from build123d import *

# Parameters (mm, degrees)
SKETCH2_W           = 120.65
SKETCH2_H           = 120.65
BOSS_EXTRUDE1_DEPTH = 2.54
SKETCH3_W           = 52.07
SKETCH3_H           = 16.51
SKETCH3_W_2         = 0.635
SKETCH3_H_2         = 6.35
SKETCH3_H_3         = 27.94
SKETCH3_W_3         = 23.495
SKETCH3_H_4         = 38.1
BOSS_EXTRUDE2_DEPTH = 2.54
BOSS_EXTRUDE4_DEPTH = 2.54


with BuildPart() as part:
    # Sketch2 → Boss-Extrude1 (new body)
    with BuildSketch(Plane(origin=(0, 0, 0), x_dir=(1, 0, 0), z_dir=(0, 1, 0))):
        Rectangle(SKETCH2_W, SKETCH2_H)
    extrude(amount=BOSS_EXTRUDE1_DEPTH)

    # Sketch3 → Boss-Extrude2 (add)
    with BuildSketch(Plane(origin=(0, 2.54, 0), x_dir=(1, 0, 0), z_dir=(0, 1, 0))):
        with Locations((-28.575, 52.07)):
            Rectangle(SKETCH3_W, SKETCH3_H)
        with Locations((-60.0075, -21.59)):
            Rectangle(SKETCH3_W_2, SKETCH3_H_2)
        with Locations((60.0075, -46.355)):
            Rectangle(SKETCH3_W_2, SKETCH3_H_3)
        with Locations((-42.8625, -21.59)):
            Rectangle(SKETCH3_W_3, SKETCH3_H_2)
        with Locations((-14.2875, -21.59)):
            Rectangle(SKETCH3_W_3, SKETCH3_H_2)
        with Locations((-60.0075, 52.07)):
            Rectangle(SKETCH3_W_2, SKETCH3_H)
        with Locations((60.0075, 5.715)):
            Rectangle(SKETCH3_W_2, SKETCH3_H_4)
        with Locations((42.8625, -21.59)):
            Rectangle(SKETCH3_W_3, SKETCH3_H_2)
        with Locations((14.2875, -21.59)):
            Rectangle(SKETCH3_W_3, SKETCH3_H_2)
        with Locations((-60.0075, 5.715)):
            Rectangle(SKETCH3_W_2, SKETCH3_H_4)
        with Locations((-60.0075, -46.355)):
            Rectangle(SKETCH3_W_2, SKETCH3_H_3)
        with Locations((60.0075, 52.07)):
            Rectangle(SKETCH3_W_2, SKETCH3_H)
        with Locations((28.575, 52.07)):
            Rectangle(SKETCH3_W, SKETCH3_H)
        with Locations((-28.575, -46.355)):
            Rectangle(SKETCH3_W, SKETCH3_H_3)
        with Locations((28.575, -46.355)):
            Rectangle(SKETCH3_W, SKETCH3_H_3)
        with Locations((60.0075, -21.59)):
            Rectangle(SKETCH3_W_2, SKETCH3_H_2)
        with Locations((28.575, 5.715)):
            Rectangle(SKETCH3_W, SKETCH3_H_4)
        with Locations((-42.8625, 35.56)):
            Rectangle(SKETCH3_W_3, SKETCH3_H_2)
        with Locations((-14.2875, 35.56)):
            Rectangle(SKETCH3_W_3, SKETCH3_H_2)
        with Locations((14.2875, 35.56)):
            Rectangle(SKETCH3_W_3, SKETCH3_H_2)
        with Locations((42.8625, 35.56)):
            Rectangle(SKETCH3_W_3, SKETCH3_H_2)
        with Locations((-28.575, 5.715)):
            Rectangle(SKETCH3_W, SKETCH3_H_4)
        with Locations((-60.0075, 35.56)):
            Rectangle(SKETCH3_W_2, SKETCH3_H_2)
        with Locations((60.0075, 35.56)):
            Rectangle(SKETCH3_W_2, SKETCH3_H_2)
    extrude(amount=BOSS_EXTRUDE2_DEPTH)

    # Sketch5 → Boss-Extrude4 (add)
    with BuildSketch(Plane(origin=(60.325, 0, 0), x_dir=(0, 0, -1), z_dir=(1, 0, 0))):
        Polygon((-60.325, 0), (60.325, 0), (60.325, 5.08), (43.815, 5.08), (43.815, 2.54), (38.735, 2.54), (38.735, 5.08), (32.385, 5.08), (32.385, 2.54), (24.765, 2.54), (24.765, 5.08), (-13.335, 5.08), (-13.335, 2.54), (-18.415, 2.54), (-18.415, 5.08), (-24.765, 5.08), (-24.765, 2.54), (-32.385, 2.54), (-32.385, 5.08), (-60.325, 5.08), align=None)
    boss_extrude4 = extrude(amount=BOSS_EXTRUDE4_DEPTH)

    # Mirror2: Boss-Extrude4 across plane
    add(boss_extrude4.mirror(Plane(origin=(0, 0, 0), x_dir=(0, 0, 1), z_dir=(1, 0, 0))))


solid = part.part
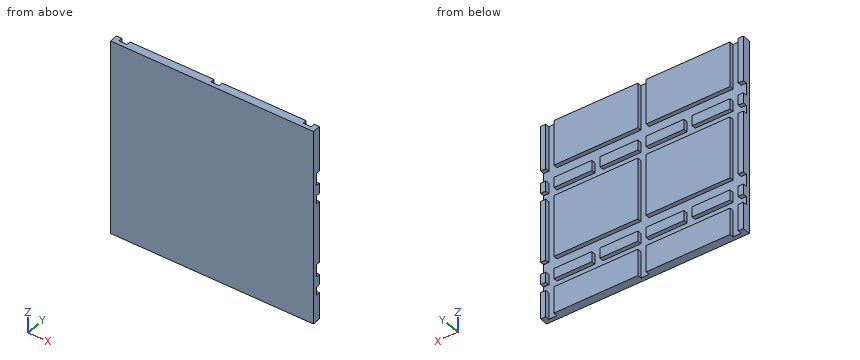
The model under review builds one solid part; all positions refer to its coordinate system, in mm. Coordinates: 2 decimals unless noted, no trailing zeros. Write each loop counter-clockwise with the first axis right and the second up, starting at its lowest first coordinate (ties: lowest second). Pieces come first, ordered by that corner, then holes. Notation, with made-up numbers: (53, 59.25) - (69, 59.25) arc R21 ccw to (69, 76.25) - close; hole circle Ø11 at (44.25, 58). An arc over 180 degrees is marked (long way). Answer as a JSON object with one key per item and string values. Group by question number.
1. Add section A-A (z = 20). Give the boundary of the cut face in (x, y) (3 decimals), plus the area to 3 significant figures.
2. Add section D-D (z = -22). Give the boundary of the cut face in (x, y) (3 decimals), plus the area to 3 significant figures.
3. Add section B-B (y = 3.7). Give the number of separate pieces and of enclosed holes in the cut face, plus the area to 3 significant figures.
4. Add section C-C (x = 33.5). Give the boundary of the cut face in (y, z) (3 decimals), plus the area to 3 significant figures.
5. To check wall thickness, follow probe 1 along X at (y, z) = (3.95, -3) (3 decimals); probe 2 along Z at (x, y) = (45.5, 2.9) (3 decimals); probe 3 along Y at (x, z) = (25.5, -26). State the ranges of each line that lie inside material, in increasing order.
Findings:
{
 "1": {"outline": "(-62.865, 0) - (62.865, 0) - (62.865, 5.08) - (59.69, 5.08) - (59.69, 2.54) - (54.61, 2.54) - (54.61, 5.08) - (31.115, 5.08) - (31.115, 2.54) - (26.035, 2.54) - (26.035, 5.08) - (2.54, 5.08) - (2.54, 2.54) - (-2.54, 2.54) - (-2.54, 5.08) - (-26.035, 5.08) - (-26.035, 2.54) - (-31.115, 2.54) - (-31.115, 5.08) - (-54.61, 5.08) - (-54.61, 2.54) - (-59.69, 2.54) - (-59.69, 5.08) - (-62.865, 5.08) - close", "area": "574 mm²"},
 "2": {"outline": "(-62.865, 0) - (62.865, 0) - (62.865, 5.08) - (59.69, 5.08) - (59.69, 2.54) - (54.61, 2.54) - (54.61, 5.08) - (2.54, 5.08) - (2.54, 2.54) - (-2.54, 2.54) - (-2.54, 5.08) - (-54.61, 5.08) - (-54.61, 2.54) - (-59.69, 2.54) - (-59.69, 5.08) - (-62.865, 5.08) - close", "area": "600 mm²"},
 "3": {"separate pieces": "24", "enclosed holes": "0", "area": "10,400 mm²"},
 "4": {"outline": "(0, -60.325) - (5.08, -60.325) - (5.08, -43.815) - (2.54, -43.815) - (2.54, -38.735) - (5.08, -38.735) - (5.08, -32.385) - (2.54, -32.385) - (2.54, -24.765) - (5.08, -24.765) - (5.08, 13.335) - (2.54, 13.335) - (2.54, 18.415) - (5.08, 18.415) - (5.08, 24.765) - (2.54, 24.765) - (2.54, 32.385) - (5.08, 32.385) - (5.08, 60.325) - (0, 60.325) - close", "area": "548 mm²"},
 "5": {"probe 1": "-62.865 to -59.69, -54.61 to -2.54, 2.54 to 54.61, 59.69 to 62.865", "probe 2": "-60.325 to -43.815, -38.735 to -32.385, -24.765 to 13.335, 18.415 to 24.765, 32.385 to 60.325", "probe 3": "0 to 2.54"}
}
